Autodesk Inventor part; units mm, degrees
ref_plane "YZ Plane" through (0, 0, 0) normal (1, 0, 0) x (0, 1, 0)
ref_plane "XZ Plane" through (0, 0, 0) normal (0, 1, 0) x (-1, 0, 0)
ref_plane "XY Plane" through (0, 0, 0) normal (0, 0, 1) x (1, 0, 0)
sketch "Sketch1" plane through (0, 0, 0) normal (0, 1, 0) x (-1, 0, 0)
  circle A0 centre (0, 0) radius 15.175
  circle A1 centre (0, 0) radius 15.7084
  dimension "d1" = 30.35
  dimension "d2" = 31.4168
extrude "Extrusion1" add sketch "Sketch1" along normal blind 110
sketch "Sketch3" plane through (0, 0, 0) normal (0, 0, 1) x (1, 0, 0)
  line L0 (15.7084, 42) -> (15.7084, 68)
  line L1 (15.7084, 68) -> (5.7084, 68)
  line L2 (5.7084, 68) -> (5.7084, 42)
  line L3 (15.7084, 42) -> (5.7084, 42)
  point P0 (0, 0)
  dimension "d7" = 26
  dimension "d8" = 10
extrude "Extrusion2" cut sketch "Sketch3" along normal mid plane 110
properties part number "DPLX_P007_Wire_Mesh_Sleeve_Spark_Gap" material "Stucco"
Source: CAD feature listing. Evaluate the final solid. Frame: model axes, mm. Give positions to 0.01 mm unless a question says otherwise; leave off trailing zeros. Loops run counter-clockwise (first coordinate to the right, second up) from the corner with the lowest first, then second, coordinate; pieces in that order, holes last. Notation, with made-up numbers: (57, -35) - (108, -35) arc R24 cw to (108, -13) - close; hole circle Ø1 at (59, 83.5). An arc over 180 degrees is marked (long way). Use CSV: the item, a comma, the result in double quotes.
1) Cut plane C-C (x = 11). Output: boundary loops of the cut face in (y, z), and give its area (3 significant figures).
Worked out:
outline,"(0, -11.21) - (42, -11.21) - (42, -10.45) - (0, -10.45) - close; (0, 10.45) - (42, 10.45) - (42, 11.21) - (0, 11.21) - close; (68, -11.21) - (110, -11.21) - (110, -10.45) - (68, -10.45) - close; (68, 10.45) - (110, 10.45) - (110, 11.21) - (68, 11.21) - close"
area,"128 mm^2"
2) Pin query (flat end, axial travel): P1, Ø8, axis at x = 10, z = -2, coming from the +Y side; P2, Ø3, axis at y = 25.5, z = 3.5, coming from the -X side; P3, Ø1, axis at y = 93.5, z = 11, coming from the -X side; P4, Ø1, axis at y = 32, z = 9, coming from the +X side. Return the tip coordinate at first contact, or that it passes through.
Worked out:
P1,"passes through"
P2,"stops at x = -15.58"
P3,"stops at x = -11.68"
P4,"stops at x = 13.21"
3) Mould query, pull axis Z, two halves, no side actions, for faces 1 (the flat face through (15.5, 68, -0.1)), 2 (the cylindrical face through (-14.51, 54.23, 6.02)), 3 (the cylindrical face through (-14.474, 54.23, -4.558)). Classes: +Z half, -Z half, draft (parallel to the pull), parting line (faces both ways), or undercut.
Worked out:
face 1,"draft"
face 2,"parting line"
face 3,"undercut"
4) Cut plane A-A (z = 0). Output: boundary loops of the cut face in (x, y) (3 decimals), and give its area (3 significant figures).
Worked out:
outline,"(-15.708, 0) - (-15.175, 0) - (-15.175, 110) - (-15.708, 110) - close; (15.175, 0) - (15.708, 0) - (15.708, 42) - (15.175, 42) - close; (15.175, 68) - (15.708, 68) - (15.708, 110) - (15.175, 110) - close"
area,"103 mm^2"
5) Cut plane D-D (y = 11). Output: boundary loops of the cut face in (x, z) (3 decimals), and give its area (3 significant figures).
Worked out:
outline,"circle Ø31.417 at (0, 0); hole circle Ø30.35 at (0, 0)"
area,"51.8 mm^2"
6) Line query: line 1 (Z direction, x = 0, y = 81) (3 decimals); line 2 (Z direction, x = -4, y = 40). Output: solid intervals per line, ascending.
Worked out:
line 1,"z = -15.708 to -15.175, 15.175 to 15.708"
line 2,"z = -15.19 to -14.64, 14.64 to 15.19"
7) Cut plane B-B (x = 0). Output: boundary loops of the cut face in (y, z) (3 decimals), and give its area (3 significant figures).
Worked out:
outline,"(0, -15.708) - (110, -15.708) - (110, -15.175) - (0, -15.175) - close; (0, 15.175) - (110, 15.175) - (110, 15.708) - (0, 15.708) - close"
area,"117 mm^2"
